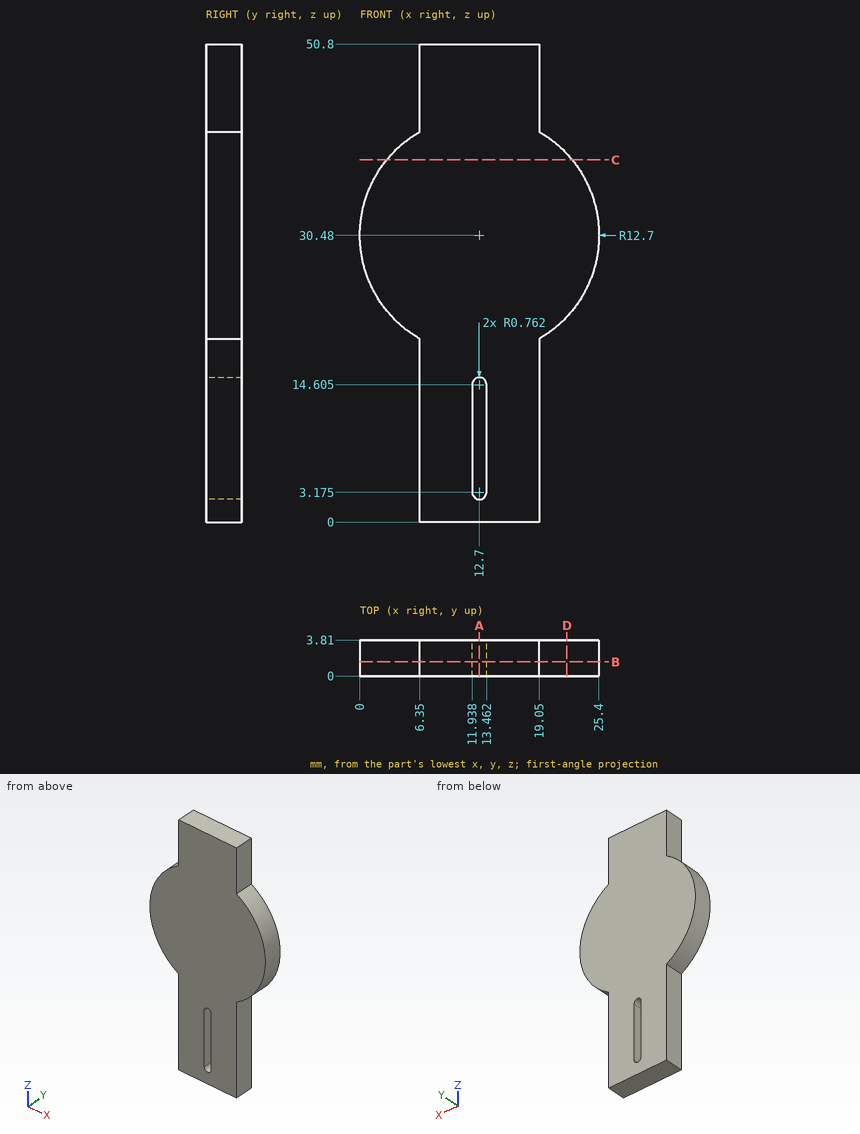
The figure shows three views and two pictorial views of one solid part (mm, origin at its lowest corner). Answer the questions. Coordinates: 2 decimals unless noted, no trailing zeros. Loops run counter-clockwise (first coordinate to the right, second up) from the corner with the lowest first, then second, coordinate; pieces in that order, holes last.
1) Find section D-D on x = 22. Write down the section's boundary in (y, z), then the cut area to 3 significant figures.
2) Flat-ended cylindrical pins translate along their axes: pin 1 Ø1.9 at (y, z) = (2.5, 8.5) entering from +X; pin 2 Ø12 at (x, z) = (20.5, 6) entering from -Y; pin 3 Ø1.1 at (y, z) = (2, 11.5) entering from -X. Find the tip coordinate at first contact, or state that the pin passes through.
3) Find section B-B on y = 1.5. Write down the section's boundary in (x, z) (3 decimals), then the cut area to 3 significant figures.
4) Find the intervals of material crossed by L1, parallel to X at y = 2.5, z = 7; L2, parallel to X at y = 3.6, z = 45; L3, parallel to X at y = 0.55, z = 15, in increasing order.
5) Find section C-C on z = 38.5. Write down the section's boundary in (x, y).
6) Find section A-A on x = 12.7. Write down the section's boundary in (y, z).
Values:
1. outline: (0, 21.83) - (3.81, 21.83) - (3.81, 39.13) - (0, 39.13) - close
1. area: 65.9 mm2
2. pin 1: stops at x = 19.05
2. pin 2: stops at y = 0
2. pin 3: stops at x = 6.35
3. outline: (6.35, 0) - (19.05, 0) - (19.05, 19.481) arc R12.7 ccw to (19.05, 41.479) - (19.05, 50.8) - (6.35, 50.8) - (6.35, 41.479) arc R12.7 ccw to (6.35, 19.481) - close; hole (11.938, 3.175) arc R0.762 ccw to (13.462, 3.175) - (13.462, 14.605) arc R0.762 ccw to (11.938, 14.605) - close
3. area: 824 mm2
4. L1: x = 6.35 to 11.94, 13.46 to 19.05
4. L2: x = 6.35 to 19.05
4. L3: x = 6.35 to 12.05, 13.35 to 19.05
5. outline: (2.85, 0) - (22.55, 0) - (22.55, 3.81) - (2.85, 3.81) - close
6. outline: (0, 0) - (3.81, 0) - (3.81, 2.41) - (0, 2.41) - close; (0, 15.37) - (3.81, 15.37) - (3.81, 50.8) - (0, 50.8) - close
